```python
from build123d import *

# Parameters (mm, degrees)
F0_R     = 21.5
F1_DEPTH = 15
F3_W     = 8
F3_H     = 10
F4_DEPTH = 10
F5_R     = 6.35
F6_DEPTH = 1


with BuildPart() as f1:
    # F0 (on Top) → F1 (new body)
    with BuildSketch(Plane.XY):
        Circle(F0_R)
    extrude(amount=F1_DEPTH)

    # F3 (on offset) → F4 (cut)
    with BuildSketch(Plane.XZ.offset(28.448)):
        with Locations((0, 7.5)):
            Rectangle(F3_W, F3_H)
    extrude(amount=-F4_DEPTH, mode=Mode.SUBTRACT)

    # F5 (on face) → F6 (cut)
    with BuildSketch(Plane(origin=(0, 0, 0), x_dir=(1, 0, 0), z_dir=(0, 0, -1))):
        Circle(F5_R)
    extrude(amount=-F6_DEPTH, mode=Mode.SUBTRACT)


solid = f1.part
```
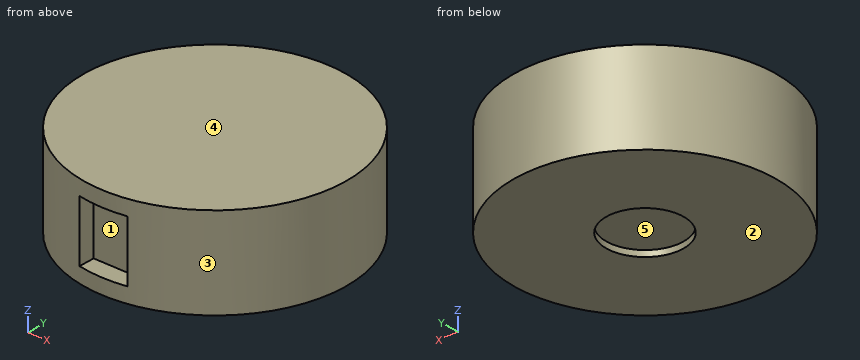
Could you check a few things on this model? Use its own coordinates, in mm. Face numbers are marked on the shaded views. A direction names the side the tool comes from. Round coordinates to 2 decimals unless told otherwise and drop trailing zeros. Loops run counter-clockwise (first coordinate to the right, second up) from the corner with the lowest first, then second, coordinate; pieces in that order, holes last. Notation, with made-up numbers: (86, -39) -> (124, -39) arc R8 cw to (124, -29) -> close; hole circle Ø4 at (68.5, 36.5). An arc over 180 degrees is marked (long way). Put each result on its own line as item: value.
Q1. I want a section at A-A on x = 0. Write out the boundary of the cut face in (y, z).
Checks:
outline: (-21.5, 0) -> (-6.35, 0) -> (-6.35, 1) -> (6.35, 1) -> (6.35, 0) -> (21.5, 0) -> (21.5, 15) -> (-21.5, 15) -> (-21.5, 12.5) -> (-18.45, 12.5) -> (-18.45, 2.5) -> (-21.5, 2.5) -> close
Q2. For pin 1 Ø4 at (x, z) = (-5, 12) entering from -Y; pin 2 Ø1.5 at (x, z) = (-5, 8) entering from -Y; pin 3 Ø3 at (y, z) = (2, 4) entering from -X, each with a flat end and sliding along its axis, tell me the tip position at first contact or that it passes through.
Checks:
pin 1: y = -21.28
pin 2: y = -21.08
pin 3: x = -21.49
Q3. Please list where these lines run through material, in increasing order: line 1 (Y direction, x = 0, z = 0.4); line 2 (Y direction, x = 0.5, z = 6); line 3 (X direction, y = -14, z = 11.5). Write a range as from..to.
Checks:
line 1: -21.5..-6.35, 6.35..21.5
line 2: -18.45..21.49
line 3: -16.32..16.32
Q4. Thinking about a two-plate mould opening in X: for the marked faces 3, 4 and 5, which applies, pulls with the +X half, pulls with the -X half, needs draft (parallel to the pull), parting line crosses it, or undercut?
Checks:
face 3: parting line crosses it
face 4: needs draft
face 5: undercut
Q5. I want a section at D-D on x = -5. Write out the boundary of the cut face in (y, z), and give its area (3 significant figures).
Checks:
outline: (-20.91, 0) -> (-3.91, 0) -> (-3.91, 1) -> (3.91, 1) -> (3.91, 0) -> (20.91, 0) -> (20.91, 15) -> (-20.91, 15) -> close
area: 619 mm2
Q6. I want a section at C-C on z = 5.25. Write out the boundary of the cut face in (x, y).
Checks:
outline: (-4, -21.12) -> (-4, -18.45) -> (4, -18.45) -> (4, -21.12) arc R21.5 ccw (long way) to start
Q7. Which directions (+Z, -Z, +X, -X, +Y, -Y) give clear straight access to the entire face, cutting with the end or side of a thin tool? Please do the marked faces 1 and 2.
Checks:
face 1: -Y
face 2: -Z, +X, -X, +Y, -Y
Q8. I want a section at B-B on y = 0. Write out the boundary of the cut face in (x, z), and give its area (3 significant figures).
Checks:
outline: (-21.5, 0) -> (-6.35, 0) -> (-6.35, 1) -> (6.35, 1) -> (6.35, 0) -> (21.5, 0) -> (21.5, 15) -> (-21.5, 15) -> close
area: 632 mm2
